Work out the finished part from the listing and answer in its coordinate system (mm). Face numbers are marked on the shaded views. A direction names the side the tool comes from. Coordinates: 2 decimals unless noted, no trailing zeros. Write each loop counter-clockwise with the first axis right and the second up, starting at its lowest first coordinate (ties: lowest second). Pieces come first, ordered by that corner, then holes. Notation, with made-up numbers: (17, 44.5) - (54, 44.5) arc R20 ccw to (54, 68.5) - close; hole circle Ø3 at (-11.5, -39). An arc over 180 degrees is marked (long way). Use a Markdown table: item, result. Add a question column.
(1) The part is cut by section C-C, the plane x = 0. Give the vertices of the cut face in (y, z), then the cut area to 3 significant figures.
(2) For a pull along Z with two mould halves and no side action, classify the marked faces 3, 4 and 5 as released by +Z, released by -Z, zero draft, split by the parting line, or undercut.
(3) Find the intervals of material crossed by line 1 (Z direction, x = 0, y = -1.4); line 2 (X direction, y = -0.45, z = 3); line 3 (Y direction, x = -1.25, z = 7.75), in increasing order. Write a range as from..to.
(4) The part is cut by section D-D, the plane z = 2.75. Give the vertices of the cut face in (x, y).
(5) The part is cut by section A-A, the plane y = -0.15. Give the vertices of the cut face in (x, z).
(6) The part is cut by section B-B, the plane z = 20. Give the vertices of the cut face in (x, y), then the cut area to 3 significant figures.
(7) A tool of negligible diameter and unlimited length cuts with its end or side. For the marked faces 1 and 2, from which of +Z, -Z, +X, -X, +Y, -Y can it reach the whole face along a straight path? Write none if from no direction.
from build123d import *

# Parameters (mm, degrees)
CROQUIS1_W              = 9
CROQUIS1_H              = 5
SALIENTE_EXTRUIR1_DEPTH = 24
CROQUIS2_W              = 7.5
CROQUIS2_H              = 3.5
CORTAR_EXTRUIR1_DEPTH   = 9
CROQUIS3_R              = 2.25
CORTAR_EXTRUIR2_DEPTH   = 9


with BuildPart() as part:
    # Croquis1 → Saliente-Extruir1 (new body)
    with BuildSketch(Plane.XY):
        Rectangle(CROQUIS1_W, CROQUIS1_H)
    extrude(amount=SALIENTE_EXTRUIR1_DEPTH)

    # Croquis2 → Cortar-Extruir1 (cut)
    with BuildSketch(Plane(origin=(0, 0, 0), x_dir=(-1, 0, 0), z_dir=(0, 0, -1))):
        Rectangle(CROQUIS2_W, CROQUIS2_H)
    extrude(amount=-CORTAR_EXTRUIR1_DEPTH, mode=Mode.SUBTRACT)

    # Croquis3 → Cortar-Extruir2 (cut)
    with BuildSketch(Plane(origin=(0, 2.5, 0), x_dir=(1, 0, 0), z_dir=(0, 1, 0))):
        with Locations(Location((0, -20, 0), (0, 0, 180))):
            Circle(CROQUIS3_R)
    extrude(amount=-CORTAR_EXTRUIR2_DEPTH, mode=Mode.SUBTRACT)


solid = part.part
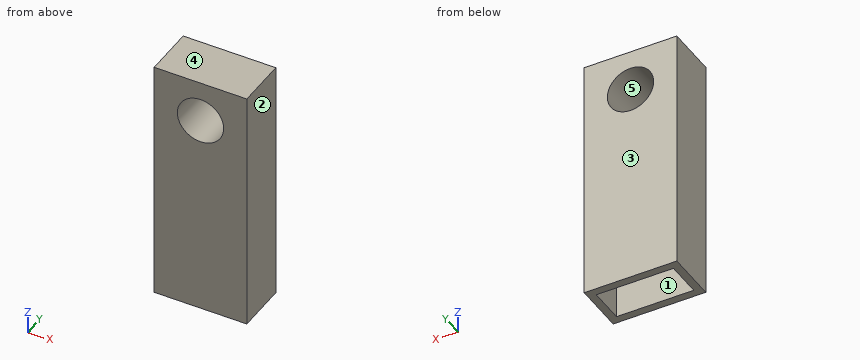
Model answer:
| question | item | result |
|---|---|---|
| 1 | outline | (-2.5, 0) - (-1.75, 0) - (-1.75, 9) - (1.75, 9) - (1.75, 0) - (2.5, 0) - (2.5, 17.75) - (-2.5, 17.75) - close; (-2.5, 22.25) - (2.5, 22.25) - (2.5, 24) - (-2.5, 24) - close |
| 1 | area | 66.0 mm^2 |
| 2 | face 3 | zero draft |
| 2 | face 4 | released by +Z |
| 2 | face 5 | undercut |
| 3 | line 1 | 9..17.75, 22.25..24 |
| 3 | line 2 | -4.5..-3.75, 3.75..4.5 |
| 3 | line 3 | -2.5..-1.75, 1.75..2.5 |
| 4 | outline | (-4.5, -2.5) - (4.5, -2.5) - (4.5, 2.5) - (-4.5, 2.5) - close; hole (-3.75, -1.75) - (3.75, -1.75) - (3.75, 1.75) - (-3.75, 1.75) - close |
| 5 | outline | (-4.5, 0) - (-3.75, 0) - (-3.75, 9) - (3.75, 9) - (3.75, 0) - (4.5, 0) - (4.5, 24) - (-4.5, 24) - close; hole circle Ø4.5 at (0, 20) |
| 6 | outline | (-4.5, -2.5) - (-2.25, -2.5) - (-2.25, 2.5) - (-4.5, 2.5) - close; (2.25, -2.5) - (4.5, -2.5) - (4.5, 2.5) - (2.25, 2.5) - close |
| 6 | area | 22.5 mm^2 |
| 7 | face 1 | -Z |
| 7 | face 2 | +Z, -Z, +X, +Y, -Y |
